from build123d import *

# Parameters (mm, degrees)
SKETCH_1_W      = 55.5
SKETCH_1_H      = 20
SKETCH_1_R      = 3
SKETCH_1_R_2    = 1.5
EXTRUDE_1_DEPTH = 2
SKETCH_2_R      = 4
SKETCH_2_R_2    = 1.1
EXTRUDE_2_DEPTH = 2
FILLET_1_R      = 2


with BuildPart() as part:
    # 草图1 → 凸台-拉伸1 (new body)
    with BuildSketch(Plane.XY):
        Rectangle(SKETCH_1_W, SKETCH_1_H)
        Circle(SKETCH_1_R, mode=Mode.SUBTRACT)
        with Locations((-4.949747468, 4.949747468)):
            Circle(SKETCH_1_R_2, mode=Mode.SUBTRACT)
        with Locations((4.949747468, 4.949747468)):
            Circle(SKETCH_1_R_2, mode=Mode.SUBTRACT)
        with Locations((4.949747468, -4.949747468)):
            Circle(SKETCH_1_R_2, mode=Mode.SUBTRACT)
        with Locations((-4.949747468, -4.949747468)):
            Circle(SKETCH_1_R_2, mode=Mode.SUBTRACT)
    extrude(amount=EXTRUDE_1_DEPTH)

    # 草图2 → 凸台-拉伸2 (add)
    with BuildSketch(Plane.ZY.offset(27.75)):
        with BuildLine():
            Line((2, 10), (2, -10))
            Line((2, -10), (22, -10))
            ThreePointArc((22, -10), (32, 0), (22, 10))
            Line((22, 10), (2, 10))
        make_face()
        with Locations(Location((22, 0, 0), (0, 0, 270))):
            Circle(SKETCH_2_R, mode=Mode.SUBTRACT)
        with Locations(Location((29, 0, 0), (0, 0, 270))):
            Circle(SKETCH_2_R_2, mode=Mode.SUBTRACT)
        with Locations(Location((22, -7, 0), (0, 0, 270))):
            Circle(SKETCH_2_R_2, mode=Mode.SUBTRACT)
        with Locations(Location((15, 0, 0), (0, 0, 270))):
            Circle(SKETCH_2_R_2, mode=Mode.SUBTRACT)
        with Locations(Location((22, 7, 0), (0, 0, 270))):
            Circle(SKETCH_2_R_2, mode=Mode.SUBTRACT)
    extrude_2 = extrude(amount=-EXTRUDE_2_DEPTH)

    # 镜向1: 凸台-拉伸2 across plane
    add(extrude_2.mirror(Plane(origin=(0, 0, 0), x_dir=(0, 0, 1), z_dir=(1, 0, 0))))

    # 圆角1
    fillet_1_edges = [part.edges().sort_by_distance(p)[0] for p in [
        (-27.75, 0, 0),
        (27.75, 0, 0),
    ]]
    fillet(fillet_1_edges, radius=FILLET_1_R)


solid = part.part
Verification items for the finished model (mm, model axes). A direction names the side the tool comes from. Give positions to 0.01 mm unless a question says otherwise; leave off trailing zeros. Loops run counter-clockwise (first coordinate to the right, second up) from the corner with the lowest first, then second, coordinate; pieces in that order, holes last.
1. Tool access check on faces 5 (the flat face through (-25.75, 0, 17)), 6 (the cylindrical face through (27.18, 0.14, 0.6)). Record the directions out of +Z, -Z, +X, -X, +Y, -Y that give a thin tool (end or side, any length) a straight path to the whole face; none if there is none.
Derived:
face 5: +Z, +Y, -Y
face 6: -Z, +X, +Y, -Y
2. Cross-section at B-B on z = 3.5. Record the cut outline in (x, y), and give its area (3 significant figures).
Derived:
outline: (-27.75, -10) - (-25.75, -10) - (-25.75, 10) - (-27.75, 10) - close; (25.75, -10) - (27.75, -10) - (27.75, 10) - (25.75, 10) - close
area: 80.0 mm2
3. Cross-section at A-A on z = 15. Record the cut outline in (x, y).
Derived:
outline: (-27.75, -10) - (-25.75, -10) - (-25.75, -1.1) - (-27.75, -1.1) - close; (-27.75, 1.1) - (-25.75, 1.1) - (-25.75, 10) - (-27.75, 10) - close; (25.75, -10) - (27.75, -10) - (27.75, -1.1) - (25.75, -1.1) - close; (25.75, 1.1) - (27.75, 1.1) - (27.75, 10) - (25.75, 10) - close
4. Cross-section at C-C on x = 0. Record the cut outline in (y, z).
Derived:
outline: (-10, 0) - (-3, 0) - (-3, 2) - (-10, 2) - close; (3, 0) - (10, 0) - (10, 2) - (3, 2) - close
5. Cross-section at D-D on y = -7. Record the cut outline in (x, z).
Derived:
outline: (-27.75, 2) arc R2 ccw to (-25.75, 0) - (25.75, 0) arc R2 ccw to (27.75, 2) - (27.75, 20.9) - (25.75, 20.9) - (25.75, 2) - (-25.75, 2) - (-25.75, 20.9) - (-27.75, 20.9) - close; (-27.75, 23.1) - (-25.75, 23.1) - (-25.75, 29.14) - (-27.75, 29.14) - close; (25.75, 23.1) - (27.75, 23.1) - (27.75, 29.14) - (25.75, 29.14) - close
6. Material ranges on probe 1 along X at (y, z) = (6.25, 18); probe 2 along Z at (x, y) = (-26.55, 0); probe 3 along Z at (x, y) = (-26.15, 0), recorded low to high.
Derived:
probe 1: x = -27.75 to -25.75, 25.75 to 27.75
probe 2: z = 0.17 to 13.9, 16.1 to 18, 26 to 27.9, 30.1 to 32
probe 3: z = 0.04 to 13.9, 16.1 to 18, 26 to 27.9, 30.1 to 32
7. Release check for a two-part mould opening along Z. For faces 1 (the cylindrical face through (-26.764, 7.238, 20.926)), 2 (the flat face through (27.75, 0, 17)), 3 (the cylindrical face through (-26.764, 0.238, 27.926)), 4 (the cylindrical face through (-27, 0, 32)) record: +Z half, -Z half, draft (parallel to the pull), parting line (faces both ways), or undercut.
Derived:
face 1: undercut
face 2: draft
face 3: undercut
face 4: +Z half
8. Go/stop test with flat-tipped pins: P1, Ø6.5, axis at y = 0, z = 22, coming from the -X side; P2, Ø3.5, axis at x = 4.95, y = -4.95, coming from the +Z side. Record where each tip stops, or that it passes through.
Derived:
P1: passes through
P2: stops at z = 2
